from build123d import *

# Parameters (mm, degrees)
EXTRUDE_1_DEPTH       = 3
EXTRUDE_START         = -3
SKETCH_2_W            = 40
SKETCH_2_H            = 6
EXTRUDE_2_DEPTH       = 3
EXTRUDE_3_DEPTH       = 3
EXTRUDE_4_DEPTH       = 3
CUT_EXTRUDE_1_DEPTH   = 10
SKETCH_7_W            = 12
SKETCH_7_H            = 4
EXTRUDE_5_DEPTH       = 3
SKETCH_8_R            = 1.05
CUT_EXTRUDE_2_DEPTH   = 10
SKETCH_9_W            = 26
SKETCH_9_H            = 6
EXTRUDE_6_DEPTH       = 3
SKETCH_10_R           = 1.6
CUT_EXTRUDE_3_DEPTH   = 10
SKETCH_14_W           = 18
SKETCH_14_H           = 6
EXTRUDE_7_DEPTH       = 3
SKETCH_15_R           = 1.6
CUT_EXTRUDE_4_DEPTH   = 10
FILLET_2_R            = 3
FILLET_3_R            = 3
FILLET_4_R            = 3
FILLET_5_R            = 10
FILLET_6_R            = 1.1
CUT_EXTRUDE_7_DEPTH   = 10
FILLET_8_R            = 2
SKETCH_17_W           = 5.387301628
SKETCH_17_H           = 6
CUT_EXTRUDE_8_DEPTH   = 10
SKETCH_18_W           = 31
SKETCH_18_H           = 6
EXTRUDE_8_DEPTH       = 3
SKETCH_19_R           = 1.6
CUT_EXTRUDE_9_DEPTH   = 10
OTHER_1_OUTLINE_R     = 1.7
OTHER_1_OUTLINE_R_2   = 1.6
OTHER_1_DEPTH         = 1.5
OTHER_1_DRAFT         = -45
OTHER_1_2_OUTLINE_R   = 1.7
OTHER_1_2_OUTLINE_R_2 = 1.6
OTHER_1_2_DEPTH       = 1.5
OTHER_1_2_DRAFT       = -45
SKETCH_23_W           = 5
SKETCH_23_H           = 6
CUT_EXTRUDE_10_DEPTH  = 10
FILLET_9_R            = 5


# Read off the part's stored shape, not the designer's step: 高级异型孔1
with BuildPart() as part:
    # 草图1 → 凸台-拉伸1 (new body)
    with BuildSketch(Plane.XY):
        with BuildLine():
            Line((0, -28.112698372), (10, -28.112698372))
            Line((10, -28.112698372), (10, -34.112698372))
            Line((10, -34.112698372), (0, -34.112698372))
            ThreePointArc((0, -34.112698372), (-24.121320344, -24.121320344), (-34.112698372, 0))
            Line((-34.112698372, 0), (-34.112698372, 20))
            Line((-34.112698372, 20), (-28.112698372, 20))
            Line((-28.112698372, 20), (-28.112698372, 0))
            ThreePointArc((-28.112698372, 0), (-19.878679656, -19.878679656), (0, -28.112698372))
        make_face()
    extrude(amount=EXTRUDE_1_DEPTH)

    # 草图2 → 凸台-拉伸2 (add)
    with BuildSketch(Plane.XY.offset(3).offset(EXTRUDE_START)):
        with BuildLine():
            Line((-24.121320344, -24.121320344), (-24.121320344, -54.112698372))
            Line((-24.121320344, -54.112698372), (-40, -54.112698372))
            Line((-40, -54.112698372), (-40, -60.112698372))
            Line((-40, -60.112698372), (10, -60.112698372))
            Line((10, -60.112698372), (10, -54.112698372))
            Line((10, -54.112698372), (-18.121320344, -54.112698372))
            Line((-18.121320344, -54.112698372), (-18.121320344, -28.901452199))
            ThreePointArc((-18.121320344, -28.901452199), (-21.256118841, -26.680584739), (-24.121320344, -24.121320344))
        make_face()
        with Locations((-31.112698372, 17)):
            Rectangle(SKETCH_2_W, SKETCH_2_H)
    extrude(amount=EXTRUDE_2_DEPTH)

    # 草图4 → 凸台-拉伸3 (add)
    with BuildSketch(Plane(origin=(0, 0, 0), x_dir=(-1, 0, 0), z_dir=(0, 0, -1))):
        with BuildLine():
            Line((-10, -28.112698372), (-21.546473969, -9.112698372))
            Line((-21.546473969, -9.112698372), (26.59478404, -9.112698372))
            ThreePointArc((26.59478404, -9.112698372), (16.342295877, -22.874727872), (0, -28.112698372))
            Line((0, -28.112698372), (-10, -28.112698372))
        make_face()
    extrude(amount=-EXTRUDE_3_DEPTH)

    # 草图6 → 凸台-拉伸4 (add)
    with BuildSketch(Plane.XY.offset(3).offset(EXTRUDE_START)):
        with BuildLine():
            Line((10, -34.112698372), (10, -54.112698372))
            Line((10, -54.112698372), (-18.121320344, -54.112698372))
            Line((-18.121320344, -54.112698372), (-18.121320344, -28.901452199))
            ThreePointArc((-18.121320344, -28.901452199), (-9.427875393, -32.784010673), (0, -34.112698372))
            Line((0, -34.112698372), (10, -34.112698372))
        make_face()
    extrude(amount=EXTRUDE_4_DEPTH)

    # 草图3 → 切除-拉伸1 (cut)
    with BuildSketch(Plane(origin=(0, 0, 0), x_dir=(-1, 0, 0), z_dir=(0, 0, -1))):
        with BuildLine():
            Line((-3.6, -29.112698372), (-10, -29.112698372))
            Line((-10, -29.112698372), (-10, -33.112698372))
            Line((-10, -33.112698372), (-3.6, -33.112698372))
            ThreePointArc((-3.6, -33.112698372), (-2.55, -34.162698372), (-1.5, -33.112698372))
            Line((-1.5, -33.112698372), (-1.5, -29.112698372))
            ThreePointArc((-1.5, -29.112698372), (-2.55, -28.062698372), (-3.6, -29.112698372))
        make_face()
    extrude(amount=-CUT_EXTRUDE_1_DEPTH, mode=Mode.SUBTRACT)

    # 草图7 → 凸台-拉伸5 (add)
    with BuildSketch(Plane(origin=(0, 0, 0), x_dir=(-1, 0, 0), z_dir=(0, 0, -1))):
        with Locations((-12, -7.112698372)):
            Rectangle(SKETCH_7_W, SKETCH_7_H)
    extrude(amount=-EXTRUDE_5_DEPTH)

    # 草图8 → 切除-拉伸2 (cut)
    with BuildSketch(Plane(origin=(0, 0, 0), x_dir=(-1, 0, 0), z_dir=(0, 0, -1))):
        with Locations((-4.95, -9.112698372)):
            Circle(SKETCH_8_R)
        with Locations((-19.05, -9.112698372)):
            Circle(SKETCH_8_R)
    extrude(amount=-CUT_EXTRUDE_2_DEPTH, mode=Mode.SUBTRACT)

    # 草图9 → 凸台-拉伸6 (add)
    with BuildSketch(Plane(origin=(0, 0, 0), x_dir=(-1, 0, 0), z_dir=(0, 0, -1))):
        with Locations((-1.887301628, 17)):
            Rectangle(SKETCH_9_W, SKETCH_9_H)
    extrude(amount=-EXTRUDE_6_DEPTH)

    # 草图10 → 切除-拉伸3 (cut)
    with BuildSketch(Plane(origin=(0, 0, 0), x_dir=(-1, 0, 0), z_dir=(0, 0, -1))):
        with Locations((41.112698372, 17)):
            Circle(SKETCH_10_R)
        with Locations((21.112698372, 17)):
            Circle(SKETCH_10_R)
        with Locations((3.5, 17)):
            Circle(SKETCH_10_R)
        with Locations((-6.5, 17)):
            Circle(SKETCH_10_R)
    extrude(amount=-CUT_EXTRUDE_3_DEPTH, mode=Mode.SUBTRACT)

    # 草图14 → 凸台-拉伸7 (add)
    with BuildSketch(Plane(origin=(0, 0, 0), x_dir=(-1, 0, 0), z_dir=(0, 0, -1))):
        with Locations((49, -57.112698372)):
            Rectangle(SKETCH_14_W, SKETCH_14_H)
    extrude(amount=-EXTRUDE_7_DEPTH)

    # 草图15 → 切除-拉伸4 (cut)
    with BuildSketch(Plane(origin=(0, 0, 0), x_dir=(-1, 0, 0), z_dir=(0, 0, -1))):
        with Locations((43, -57.112698372)):
            Circle(SKETCH_15_R)
        with Locations((23, -57.112698372)):
            Circle(SKETCH_15_R)
    extrude(amount=-CUT_EXTRUDE_4_DEPTH, mode=Mode.SUBTRACT)

    # 圆角2
    fillet_2_edges = [part.edges().sort_by_distance(p)[0] for p in [
        (-26.59478404, -9.112698372, 1.5),
    ]]
    fillet(fillet_2_edges, radius=FILLET_2_R)

    # 圆角3
    fillet_3_edges = [part.edges().sort_by_distance(p)[0] for p in [
        (10, -28.112698372, 1.5),
    ]]
    fillet(fillet_3_edges, radius=FILLET_3_R)

    # 圆角4
    fillet_4_edges = [part.edges().sort_by_distance(p)[0] for p in [
        (10, -60.112698372, 1.5),
    ]]
    fillet(fillet_4_edges, radius=FILLET_4_R)

    # 圆角5
    fillet_5_edges = [part.edges().sort_by_distance(p)[0] for p in [
        (-24.121320344, -24.121320344, 1.5),
        (-24.121320344, -54.112698372, 1.5),
    ]]
    fillet(fillet_5_edges, radius=FILLET_5_R)

    # 圆角6
    fillet_6_edges = [part.edges().sort_by_distance(p)[0] for p in [
        (-58, -60.112698372, 1.5),
        (-58, -54.112698372, 1.5),
    ]]
    fillet(fillet_6_edges, radius=FILLET_6_R)

    # 草图16 → 切除-拉伸7 (cut)
    with BuildSketch(Plane(origin=(0, 0, 0), x_dir=(-1, 0, 0), z_dir=(0, 0, -1))):
        with BuildLine():
            Line((-4, -37.112698372), (0, -37.112698372))
            ThreePointArc((0, -37.112698372), (9.363584206, -35.912054679), (18.121320344, -32.387808346))
            Line((18.121320344, -32.387808346), (18.121320344, -54.112698372))
            Line((18.121320344, -54.112698372), (-4, -54.112698372))
            Line((-4, -54.112698372), (-4, -37.112698372))
        make_face()
        with BuildLine():
            Line((-7.142425951, -25.112698372), (0, -25.112698372))
            ThreePointArc((0, -25.112698372), (12.275023024, -21.908250256), (21.417393888, -13.112698372))
            Line((21.417393888, -13.112698372), (-14.434935826, -13.112698372))
            Line((-14.434935826, -13.112698372), (-7.142425951, -25.112698372))
        make_face()
    extrude(amount=-CUT_EXTRUDE_7_DEPTH, mode=Mode.SUBTRACT)

    # 圆角8
    fillet_8_edges = [part.edges().sort_by_distance(p)[0] for p in [
        (4, -54.112698372, 1.5),
        (4, -37.112698372, 1.5),
        (-18.121320344, -32.387808346, 1.5),
        (-18.121320344, -54.112698372, 1.5),
        (-21.417393888, -13.112698372, 1.5),
        (7.142425951, -25.112698372, 1.5),
        (14.434935826, -13.112698372, 1.5),
    ]]
    fillet(fillet_8_edges, radius=FILLET_8_R)

    # 草图17 → 切除-拉伸8 (cut)
    with BuildSketch(Plane(origin=(0, 0, 0), x_dir=(-1, 0, 0), z_dir=(0, 0, -1))):
        with Locations((-12.193650814, 17)):
            Rectangle(SKETCH_17_W, SKETCH_17_H)
    extrude(amount=-CUT_EXTRUDE_8_DEPTH, mode=Mode.SUBTRACT)

    # 草图18 → 凸台-拉伸8 (add)
    with BuildSketch(Plane(origin=(0, 0, 0), x_dir=(-1, 0, 0), z_dir=(0, 0, -1))):
        with Locations((31.612698372, 17)):
            Rectangle(SKETCH_18_W, SKETCH_18_H)
    extrude(amount=-EXTRUDE_8_DEPTH)

    # 草图19 → 切除-拉伸9 (cut)
    with BuildSketch(Plane(origin=(0, 0, 0), x_dir=(-1, 0, 0), z_dir=(0, 0, -1))):
        with Locations((21.112698372, 17)):
            Circle(SKETCH_19_R)
        with Locations((41.112698372, 17)):
            Circle(SKETCH_19_R)
    extrude(amount=-CUT_EXTRUDE_9_DEPTH, mode=Mode.SUBTRACT)


with BuildPart() as other_1_tool:
    # 高级异型孔1 outline → 高级异型孔1 (with draft: the straight prism first)
    with BuildSketch(Plane.XY.offset(1.5)):
        with Locations((-21.112698372, 17)):
            Circle(OTHER_1_OUTLINE_R)
        with Locations((-21.112698372, 17)):
            Circle(OTHER_1_OUTLINE_R_2, mode=Mode.SUBTRACT)
    extrude(amount=OTHER_1_DEPTH)
    # 高级异型孔1: the draft: its side faces are tilted about the plane it starts from
    other_1_sides = [other_1_tool.faces().sort_by_distance(p)[0] for p in [
        (-22.812698372, 17, 2.25),
        (-22.712698372, 17, 2.25),
    ]]
    draft(other_1_sides, Plane.XY.offset(1.5), OTHER_1_DRAFT)


with BuildPart() as part_1:
    add(part.part)

    # 高级异型孔1: cut by other_1_tool
    add(other_1_tool.part, mode=Mode.SUBTRACT)


with BuildPart() as other_1_2_tool:
    # Other 1 2 outline → Other 1 2 (with draft: the straight prism first)
    with BuildSketch(Plane.XY.offset(1.5)):
        with Locations((-41.112698372, 17)):
            Circle(OTHER_1_2_OUTLINE_R)
        with Locations((-41.112698372, 17)):
            Circle(OTHER_1_2_OUTLINE_R_2, mode=Mode.SUBTRACT)
    extrude(amount=OTHER_1_2_DEPTH)
    # Other 1 2: the draft: its side faces are tilted about the plane it starts from
    other_1_2_sides = [other_1_2_tool.faces().sort_by_distance(p)[0] for p in [
        (-42.812698372, 17, 2.25),
        (-42.712698372, 17, 2.25),
    ]]
    draft(other_1_2_sides, Plane.XY.offset(1.5), OTHER_1_2_DRAFT)


with BuildPart() as part_2:
    add(part_1.part)

    # Other 1 2: cut by other_1_2_tool
    add(other_1_2_tool.part, mode=Mode.SUBTRACT)

    # 草图23 → 切除-拉伸10 (cut)
    with BuildSketch(Plane(origin=(0, 0, 0), x_dir=(-1, 0, 0), z_dir=(0, 0, -1))):
        with Locations((48.612698372, 17)):
            Rectangle(SKETCH_23_W, SKETCH_23_H)
    extrude(amount=-CUT_EXTRUDE_10_DEPTH, mode=Mode.SUBTRACT)

    # 圆角9
    fillet_9_edges = [part_2.edges().sort_by_distance(p)[0] for p in [
        (-28.112698372, 14, 1.5),
        (-34.112698372, 14, 1.5),
    ]]
    fillet(fillet_9_edges, radius=FILLET_9_R)


solid = part_2.part
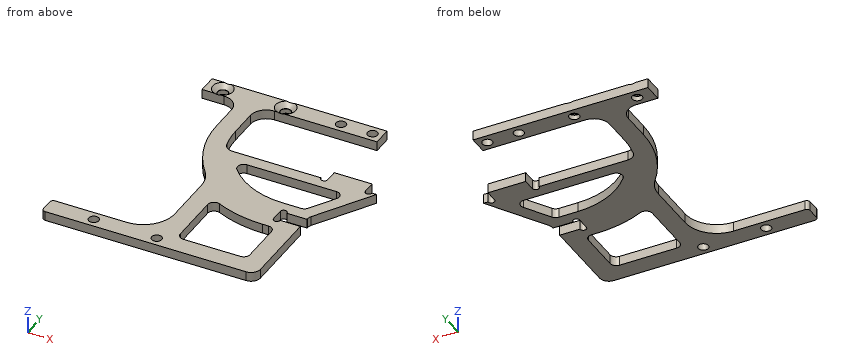
Could you check a few things on this model? Use its own coordinates, in mm. Round coordinates to 2 decimals unless told otherwise and drop trailing zeros. Write each loop counter-clockwise with the first axis right and the second up, starting at its lowest first coordinate (ties: lowest second). Pieces come first, ordered by that corner, then holes. Notation, with made-up numbers: (25, 54.25) -> (75, 54.25) arc R14 ccw to (75, 76.25) -> close; hole circle Ø3 at (-36.5, 58.5). An arc over 180 degrees is marked (long way). Use a Markdown table: item, result.
1. For pin 1 Ø0.9 at (y, z) = (15.5, 2) entering from +X; pin 2 Ø1 at (x, y) = (-24, -7) entering from +Z; pin 3 Ø1.5 at (y, z) = (-42.5, 1) entering from +X; pin 4 Ø0.9 at (x, z) = (-47.5, 2) entering from +Y, each with a flat end and sliding along its axis, tell me the tip position at first contact or that it passes through.
Answer key:
| item | result |
|---|---|
| pin 1 | stops at x = 9.5 |
| pin 2 | passes through |
| pin 3 | stops at x = 10 |
| pin 4 | stops at y = -54.11 |
2. Please list where these lines run through material, in increasing order: probe 1 along Y at (x, z) = (1, 2.1); probe 2 along Y at (x, z) = (-23, 0.8); probe 3 along Y at (x, z) = (-8.5, 2.05).
Answer key:
| item | result |
|---|---|
| probe 1 | y = -60.11 to -54.11, -37.11 to -25.11, -13.11 to -9.11, 14 to 20 |
| probe 2 | y = -60.11 to -58.71, -55.51 to -9.11, 14 to 20 |
| probe 3 | y = -60.11 to -54.11, -36.13 to -23.63, -13.11 to -9.11, 14 to 20 |
3. If we section it at B-B (x = -9.5): List the corners of the cut face in (y, z) for me, then the cut area to 3 significant figures.
Answer key:
| item | result |
|---|---|
| outline | (-60.11, 0) -> (-54.11, 0) -> (-54.11, 3) -> (-60.11, 3) -> close; (-35.88, 0) -> (-23.25, 0) -> (-23.25, 3) -> (-35.88, 3) -> close; (-13.11, 0) -> (-9.11, 0) -> (-9.11, 3) -> (-13.11, 3) -> close; (14, 0) -> (20, 0) -> (20, 3) -> (14, 3) -> close |
| area | 85.9 mm^2 |
4. If we section it at D-D (z = 0.6): State how many separate pieces and enclosed holes the cut face has, then the cut area to 3 significant figures.
Answer key:
| item | result |
|---|---|
| separate pieces | 1 |
| enclosed holes | 8 |
| area | 1,890 mm^2 |
5. If we section it at A-A (y = 17): List the corners of the cut face in (x, z) for me, then the cut area to 3 significant figures.
Answer key:
| item | result |
|---|---|
| outline | (-46.11, 0) -> (-42.71, 0) -> (-42.71, 1.5) -> (-42.81, 1.5) -> (-44.31, 3) -> (-46.11, 3) -> close; (-39.51, 0) -> (-22.71, 0) -> (-22.71, 1.5) -> (-22.81, 1.5) -> (-24.31, 3) -> (-37.91, 3) -> (-39.41, 1.5) -> (-39.51, 1.5) -> close; (-19.51, 0) -> (-5.1, 0) -> (-5.1, 3) -> (-17.91, 3) -> (-19.41, 1.5) -> (-19.51, 1.5) -> close; (-1.9, 0) -> (4.9, 0) -> (4.9, 3) -> (-1.9, 3) -> close; (8.1, 0) -> (9.5, 0) -> (9.5, 3) -> (8.1, 3) -> close |
| area | 123 mm^2 |
6. If we section it at C-C (x = -36.5): List the corners of the cut face in (y, z) for me.
Answer key:
| item | result |
|---|---|
| outline | (-60.11, 0) -> (-54.11, 0) -> (-54.11, 3) -> (-60.11, 3) -> close; (13.26, 0) -> (20, 0) -> (20, 3) -> (13.26, 3) -> close |
